from build123d import *

# Parameters (mm, degrees)
BOSS_EXTRUDE1_DEPTH          = 44.45
F_1_8_0_125_DIAMETER_HOLE1_D = 3.175
BOSS_EXTRUDE2_DEPTH          = 38.1
CUT_EXTRUDE1_DEPTH           = 541.666761283
CUT_EXTRUDE1_DEPTH_BACK      = 541.666761283
F_1_8_0_125_DIAMETER_HOLE2_D = 3.175
F_1_8_0_125_DIAMETER_HOLE3_D = 3.175
F_1_8_0_125_DIAMETER_HOLE4_D = 3.175


with BuildPart() as part:
    # Sketch1 → Boss-Extrude1 (new, symmetric)
    with BuildSketch(Plane.XY):
        Polygon((0, 0), (-208.79812848, 438.15), (-273.64947152, 438.15), (-273.64947152, 476.25), (-184.74947152, 476.25), (24.04865696, 38.1), (88.9, 38.1), (88.9, 0), align=None)
    extrude(amount=BOSS_EXTRUDE1_DEPTH, both=True)

    # 1/8 (0.125) Diameter Hole1 (through all)
    with Locations(Plane(origin=(56.47432848, 38.1, 0), x_dir=(0, 0, 1), z_dir=(0, 1, 0))):
        with Locations((0, 0)):
            Hole(F_1_8_0_125_DIAMETER_HOLE1_D / 2)

    # Sketch4 → Boss-Extrude2 (add)
    with BuildSketch(Plane(origin=(0, 476.25, 0), x_dir=(1, 0, 0), z_dir=(0, 1, 0))):
        Polygon((-247.611264367, 62.861792847), (-184.74947152, 0), (-247.611264367, -62.861792847), (-310.473057215, 0), align=None)
    extrude(amount=BOSS_EXTRUDE2_DEPTH)

    # Sketch6 → Cut-Extrude1 (cut, two sides: drawn at the far end of the back side and taken through both)
    with BuildSketch(Plane.XZ.offset(-438.15).offset(-CUT_EXTRUDE1_DEPTH_BACK)):
        Polygon((-310.473057215, 34.697981215), (-229.19947152, 0), (-310.473057215, -190.368300991), align=None)
    extrude(amount=CUT_EXTRUDE1_DEPTH + CUT_EXTRUDE1_DEPTH_BACK, mode=Mode.SUBTRACT)

    # 1/8 (0.125) Diameter Hole2 (through all)
    with Locations(Plane(origin=(-92.37473576, 0, -92.37473576), x_dir=(0.707106781186549, 0, -0.707106781186546), z_dir=(0.707106781186546, 0, 0.707106781186549))):
        with Locations((-194.137604132, 495.3)):
            Hole(F_1_8_0_125_DIAMETER_HOLE2_D / 2)

    # 1/8 (0.125) Diameter Hole3 (through all)
    with Locations(Plane(origin=(-92.37473576, 0, 92.37473576), x_dir=(-0.707106781186549, 0, -0.707106781186546), z_dir=(0.707106781186546, 0, -0.707106781186549))):
        with Locations((194.137604132, 495.3)):
            Hole(F_1_8_0_125_DIAMETER_HOLE3_D / 2)

    # 1/8 (0.125) Diameter Hole4 (through all)
    with Locations(Plane(origin=(0, 438.15, 0), x_dir=(-1, 0, 0), z_dir=(0, -1, 0))):
        with Locations((247.611264367, -25.4), (226.57812848, 25.4)):
            Hole(F_1_8_0_125_DIAMETER_HOLE4_D / 2)


solid = part.part
Could you check a few things on this model? Use its own coordinates, in mm. A direction names the side the tool comes from. Round coordinates to 2 decimals unless told otherwise and drop trailing zeros. Order: outer loops, then holes, each group sorted by start corner. A loop starts at its lowest first (then second) coordinate and runs counter-clockwise, first axis right, second up. Notation, with made-up numbers: M 3.5,57.5 L 45.5,57.5 A27 cw 45.5,78.5 Z; hole C 81.5,80.25 d4. An arc over 180 degrees is marked long. One line per item, written item: value.
(1) Imagine slicing it at A-A (z = -11). Write out the boundary of the cut face in (x, y), and give its area (3 significant figures).
Ans:
outline: M -233.9,438.15 L -208.8,438.15 L 0,0 L 88.9,0 L 88.9,38.1 L 24.05,38.1 L -184.75,476.25 L -195.75,476.25 L -195.75,514.35 L -233.9,514.35 Z
area: 24,300 mm^2
(2) If we mould it in two halves opening along Z, with no side actions, what happens to faces 5 (the flat face through (-273.649, 457, 32)), 6 (the flat face through (-92, 239, 44.45)), 7 (the flat face through (-216.62, 495.03, -31.87)), 8 (the flat face through (-241.188, 476.783, -28.08))? For each: released by +Z, released by -Z, zero draft, split by the parting line, or undercut.
Ans:
face 5: zero draft
face 6: released by +Z
face 7: released by -Z
face 8: undercut
(3) Imagine slicing it at C-C (y = 88.5). Write out the boundary of the cut face in (x, z), and give its area (3 significant figures).
Ans:
outline: M -42.17,-44.45 L 0.03,-44.45 L 0.03,44.45 L -42.17,44.45 Z
area: 3,750 mm^2
(4) I need wall thicknesses on line 1 along X through (y, z) = (467, 25); line 2 along X through (y, z) = (21, 0); line 3 along Z through (x, y) = (-9, 37). Which ranges of each line are inside material? Lowest first, please. Write a range as from..to.
Ans:
line 1: x = -273.65..-249.15, -246.07..-180.34
line 2: x = -10.01..54.89, 58.06..88.9
line 3: z = -44.45..44.45
(5) I'm going to push flat-ended pins straight in: P1, Ø8, axis at y = 144.5, z = 0, coming from the -X side; P2, Ø5, axis at y = 235, z = -6.5, coming from the +X side; P3, Ø14.5, axis at x = -248, z = 53, coming from the -Y side. Where does each tip first touch, or does it pass through?
Ans:
P1: stops at x = -70.77
P2: stops at x = -68.59
P3: stops at y = 476.25
(6) Which directions (+Z, -Z, +X, -X, +Y, -Y) give clear straight access to the entire face, cutting with the end or side of a thin tool? Please do faces 1 (the flat face through (-258.08, 476.78, 12.33)), 2 (the flat face through (-247, 476.25, 51)), 3 (the flat face through (49, 38.1, 1)), 4 (the flat face through (-215.74, 495.03, 30.99)).
Ans:
face 1: -X, +Y, -Y
face 2: +Z, +X, -X, -Y
face 3: +Z, -Z, +X, +Y
face 4: +Z, +X, +Y
(7) Imagine slicing it at B-B (x = 34). Write out the boundary of the cut face in (y, z).
Ans:
outline: M 0,-44.45 L 38.1,-44.45 L 38.1,44.45 L 0,44.45 Z
